Build history of the part. All positions in model axes, mm. Round coordinates to 2 decimals unless told otherwise and drop trailing zeros. Write each loop counter-clockwise with the first axis right and the second up, starting at its lowest first coordinate (ties: lowest second). Pieces come first, ordered by that corner, then holes.
from build123d import *

# Parameters (mm, degrees)
SKETCH1_W           = 140
SKETCH1_H           = 100
BOSS_EXTRUDE1_DEPTH = 3
SKETCH2_R           = 1.5
CUT_EXTRUDE1_DEPTH  = 4
SKETCH3_R           = 1.5
CUT_EXTRUDE2_DEPTH  = 10


with BuildPart() as part:
    # Sketch1 → Boss-Extrude1 (new body)
    with BuildSketch(Plane.XY):
        Rectangle(SKETCH1_W, SKETCH1_H)
    extrude(amount=BOSS_EXTRUDE1_DEPTH)

    # Sketch2 → Cut-Extrude1 (cut)
    with BuildSketch(Plane.XY.offset(3)):
        Circle(SKETCH2_R)
        with Locations((10, 0)):
            Circle(SKETCH2_R)
        with Locations((20, 0)):
            Circle(SKETCH2_R)
        with Locations((30, 0)):
            Circle(SKETCH2_R)
        with Locations((40, 0)):
            Circle(SKETCH2_R)
        with Locations((50, 0)):
            Circle(SKETCH2_R)
        with Locations((60, 0)):
            Circle(SKETCH2_R)
        with Locations((-10, 0)):
            Circle(SKETCH2_R)
        with Locations((-20, 0)):
            Circle(SKETCH2_R)
        with Locations((-30, 0)):
            Circle(SKETCH2_R)
        with Locations((-40, 0)):
            Circle(SKETCH2_R)
        with Locations((-50, 0)):
            Circle(SKETCH2_R)
        with Locations((-60, 0)):
            Circle(SKETCH2_R)
    extrude(amount=-CUT_EXTRUDE1_DEPTH, mode=Mode.SUBTRACT)

    # Sketch3 → Cut-Extrude2 (cut)
    with BuildSketch(Plane.XY.offset(3)):
        with Locations((50.25, -46.5)):
            Circle(SKETCH3_R)
        with Locations((-50.25, -46.5)):
            Circle(SKETCH3_R)
        with Locations((-1.25, -46.5)):
            Circle(SKETCH3_R)
        with Locations((-1.25, 11.5)):
            Circle(SKETCH3_R)
        with Locations((50.25, 11.5)):
            Circle(SKETCH3_R)
        with Locations((-50.25, 11.5)):
            Circle(SKETCH3_R)
    extrude(amount=-CUT_EXTRUDE2_DEPTH, mode=Mode.SUBTRACT)


solid = part.part
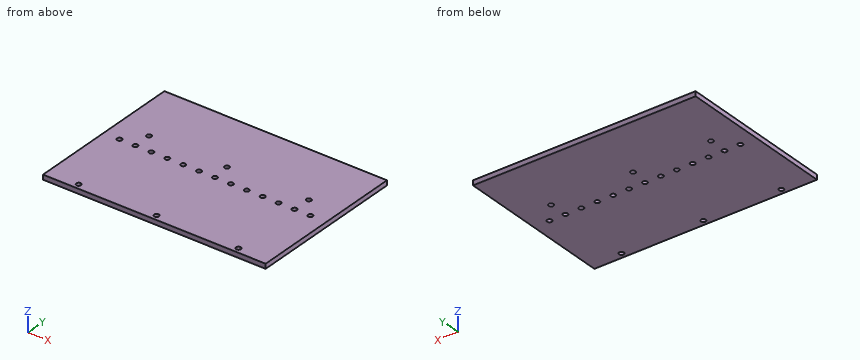
1) Slice it at A-A (x = -40). Write the cut outline in (y, z), plus the area to 3 significant figures.
Results:
outline: (-50, 0) - (-1.5, 0) - (-1.5, 3) - (-50, 3) - close; (1.5, 0) - (50, 0) - (50, 3) - (1.5, 3) - close
area: 291 mm2
2) Wall check: L1, parallel to Y at x = 50.25, z = 2.2; L2, parallel to Y at x = -30, z = 1.25; L3, parallel to Y at x = -1.25, z = 0.7. Give the ranges that are in metal, low to high.
Results:
L1: y = -50 to -48, -45 to -1.48, 1.48 to 10, 13 to 50
L2: y = -50 to -1.5, 1.5 to 50
L3: y = -50 to -48, -45 to -0.83, 0.83 to 10, 13 to 50
3) Pin check, flat tip, straight feed: pin 1 Ø3.5 at (x, y) = (0, 0) entering from +Z. Stop position of the tip, or through.
Results:
pin 1: stops at z = 3
4) Slice it at B-B (y = 0). Count the separate pieces of the cut face and the enclosed holes in it, plus the area to 3 significant figures.
Results:
separate pieces: 14
enclosed holes: 0
area: 303 mm2
